Check sheet for the modelled part. Datum: model origin and axes. Units: mm. A direction names the side the tool comes from. Give positions to 0.01 mm unless a question says otherwise; leave off trailing zeros. Loops run counter-clockwise (first coordinate to the right, second up) from the corner with the lowest first, then second, coordinate; pieces in that order, holes last. Notation, with made-up numbers: M -27,13.5 L 30,13.5 A23 ccw 30,50.5 Z; hole C 40.5,5.5 d7. An arc over 180 degrees is marked long. Use one line per item in the form item = value.
from build123d import *

# Parameters (mm, degrees)
SKETCH_1_W          = 10
SKETCH_1_H          = 15
SKETCH_1_W_2        = 7
SKETCH_1_H_2        = 12
EXTRUDE_1_DEPTH     = 771
SKETCH_2_R          = 1.5
SKETCH_2_R_2        = 2.5
SKETCH_2_R_3        = 2
CUT_EXTRUDE_1_DEPTH = 772.101322784
SKETCH_3_R          = 4
CUT_EXTRUDE_2_DEPTH = 1.5


with BuildPart() as part:
    # ｽｹｯﾁ1 → 押し出し-薄板1 (new body)
    with BuildSketch(Plane.XY):
        Rectangle(SKETCH_1_W, SKETCH_1_H)
        Rectangle(SKETCH_1_W_2, SKETCH_1_H_2, mode=Mode.SUBTRACT)
    extrude(amount=EXTRUDE_1_DEPTH)

    # ｽｹｯﾁ2 → ｶｯﾄ - 押し出し1 (cut, through all)
    with BuildSketch(Plane(origin=(5, 0, 0), x_dir=(0, 0, -1), z_dir=(1, 0, 0))):
        with Locations((-5, 4)):
            Circle(SKETCH_2_R)
        with Locations((-5, -4)):
            Circle(SKETCH_2_R)
        with Locations((-766, 4)):
            Circle(SKETCH_2_R)
        with Locations((-766, -4)):
            Circle(SKETCH_2_R)
        with Locations((-50, 0)):
            Circle(SKETCH_2_R_2)
        with Locations((-742, 0)):
            Circle(SKETCH_2_R)
        with Locations((-690, 0)):
            Circle(SKETCH_2_R_2)
        with Locations((-440, 0)):
            Circle(SKETCH_2_R_3)
        with Locations((-460, 0)):
            Circle(SKETCH_2_R_3)
        with Locations((-610, 0)):
            Circle(SKETCH_2_R_2)
        with Locations((-210, 0)):
            Circle(SKETCH_2_R_2)
    extrude(amount=-CUT_EXTRUDE_1_DEPTH, mode=Mode.SUBTRACT)

    # ｽｹｯﾁ3 → ｶｯﾄ - 押し出し2 (cut)
    with BuildSketch(Plane.ZY.offset(5)):
        with Locations((440, 0)):
            Circle(SKETCH_3_R)
        with Locations((460, 0)):
            Circle(SKETCH_3_R)
    extrude(amount=-CUT_EXTRUDE_2_DEPTH, mode=Mode.SUBTRACT)


solid = part.part
1) Scan lines: line 1 (Y direction, x = 4.35, z = 5); line 2 (Y direction, x = 1.5, z = 216.5); line 3 (X direction, y = -5, z = 287.5). Record each from-to range of solid material in increasing order.
Evaluation:
line_1 = -7.5 to -5.5, -2.5 to 2.5, 5.5 to 7.5
line_2 = -7.5 to -6, 6 to 7.5
line_3 = -5 to -3.5, 3.5 to 5
2) Depth check by flat-ended pin: pin 1 Ø3 at (y, z) = (0, 50) entering from +X; pin 2 Ø5 at (y, z) = (0, 440) entering from -X. Enter the tip coordinate at first touch or a pass-through.
Evaluation:
pin_1 = through
pin_2 = 3.5
3) Section check A-A (x = 1.5). Record the cut outline in (y, z).
Evaluation:
outline = M -7.5,0 L -6,0 L -6,771 L -7.5,771 Z; M 6,0 L 7.5,0 L 7.5,771 L 6,771 Z
4) Section check B-B (z = 314.5). Record the cut outline in (x, y), then the cut area to 3 significant figures.
Evaluation:
outline = M -5,-7.5 L 5,-7.5 L 5,7.5 L -5,7.5 Z; hole M -3.5,-6 L 3.5,-6 L 3.5,6 L -3.5,6 Z
area = 66.0 mm^2
5) Release check for a two-part mould opening along Y. For faces 3 (the face through (-3.5, 0, 380)), 4 (the face through (-5, 0, 380)) record: pulls with the +Y half, pulls with the -Y half, needs draft (parallel to the pull), parting line crosses it, or undercut.
Evaluation:
face_3 = undercut
face_4 = needs draft
6) Set-up check for faces 1 (the face through (5, 0, 380)), 2 (the face through (3.5, 0, 380)): record each of +Z, -Z, +X, -X, +Y, -Y from which the full face is reachable in a straight line by a thin tool's end or side.
Evaluation:
face_1 = +Z, -Z, +X, +Y, -Y
face_2 = +Z, -Z
